from build123d import *

# Parameters (mm, degrees)
BOX_W          = 3.2
BOX_H          = 4.2
BOX_DEPTH      = 5
CYLINDER_R     = 4
CYLINDER_DEPTH = 10


with BuildPart() as obj1:
    # Box → Box (new body)
    with BuildSketch(Plane(origin=(-1.6, -2.1, 5), x_dir=(1, 0, 0), z_dir=(0, 0, 1))):
        with Locations((1.6, 2.1)):
            Rectangle(BOX_W, BOX_H)
    extrude(amount=BOX_DEPTH)


with BuildPart() as obj2:
    # Cylinder → Cylinder (new body)
    with BuildSketch(Plane.XY):
        Circle(CYLINDER_R)
    extrude(amount=CYLINDER_DEPTH)


with BuildPart() as obj3:
    # Sphere → Sphere (revolve)
    with BuildSketch(Plane.XZ):
        with BuildLine():
            ThreePointArc((0, -5), (5, 0), (0, 5))
            Line((0, 5), (0, -5))
        make_face()
    revolve(axis=Axis((0, 0, 0), (0, 0, 1)))

    # Fusion: union obj2
    add(obj2.part)

    # Cut: cut obj1
    add(obj1.part, mode=Mode.SUBTRACT)


solid = obj3.part
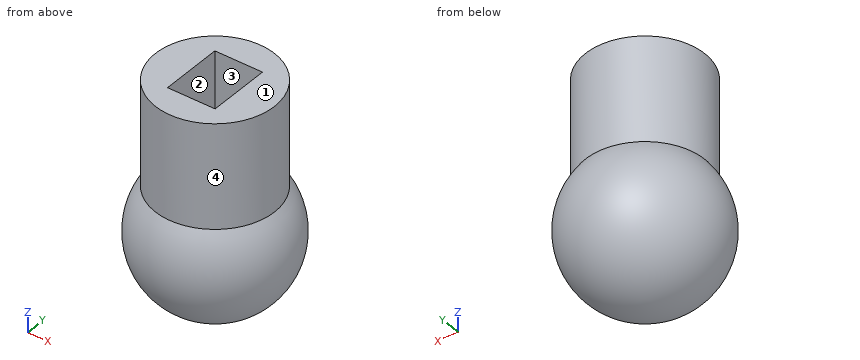
Could you check a few things on this model? Use its own coordinates, in mm. Face numbers are marked on the shaded views. Give positions to 0.01 mm unless a question says otherwise; leave off trailing zeros. Write each loop counter-clockwise with the first axis right and the second up, starting at its lowest first coordinate (ties: lowest second). Pieces come first, ordered by that corner, then holes. Notation, with made-up numbers: (-38, 41.5) - (16, 41.5) arc R13 ccw to (16, 64.5) - close; hole circle Ø2 at (-30.75, 88.25). An arc over 180 degrees is marked (long way). Use CSV: the item, a comma, the result in double quotes. Start each with the question number.
Item 1: I'm going to push flat-ended pins straight in: pin 1 (1.6 mm diameter, centred on x = 0, z = 6.5, fed in from +Y); pin 2 (5 mm diameter, centred on y = 0.5, z = 6, fed in from +X); pin 3 (1.6 mm diameter, centred on x = -0.5, z = 7.5, fed in from -Y); pin 4 (3.5 mm diameter, centred on x = 0, y = 0, fed in from +Z). Where does each tip first touch, or does it pass through?
Item 2: I want a section at B-B, the plane z = 6.75. Please give me the cut outline in (x, y), then the cut area to 3 significant figures.
Item 3: I want a section at D-D, the plane z = 0. Please give me the cut outline in (x, y), then the cut area to 3 significant figures.
Item 4: If I drill on line 1 along Y through (x, z) = (1.5, 9); line 2 along Y through (x, z) = (0, 6.75); line 3 along X through (y, z) = (1, 9.75), over which ranges is the centre line in solid material (lowest first)?
Item 5: I want a section at A-A, the plane y = 0. Please give me the cut outline in (x, z).
Item 6: If we mould it in two halves opening along X, with no side actions, what happens to the marked faces 1, 2, 3 and 4? For each: pulls with the +X half, pulls with the -X half, needs draft (parallel to the pull), parting line crosses it, or undercut.
Item 7: I want a section at C-C, the plane x = 0. Please give me the cut outline in (y, z).
Findings:
1,pin 1,"stops at y = 4"
1,pin 2,"stops at x = 4"
1,pin 3,"stops at y = -4"
1,pin 4,"stops at z = 10"
2,outline,"circle Ø8 at (0, 0); hole (-1.6, -2.1) - (1.6, -2.1) - (1.6, 2.1) - (-1.6, 2.1) - close"
2,area,"36.8 mm2"
3,outline,"circle Ø10 at (0, 0)"
3,area,"78.5 mm2"
4,line 1,"y = -3.71 to -2.1, 2.1 to 3.71"
4,line 2,"y = -4 to -2.1, 2.1 to 4"
4,line 3,"x = -3.87 to -1.6, 1.6 to 3.87"
5,outline,"(-4, 3) arc R5 ccw (long way) to (4, 3) - (4, 10) - (1.6, 10) - (1.6, 5) - (-1.6, 5) - (-1.6, 10) - (-4, 10) - close"
6,face 1,"needs draft"
6,face 2,"undercut"
6,face 3,"undercut"
6,face 4,"parting line crosses it"
7,outline,"(-4, 3) arc R5 ccw (long way) to (4, 3) - (4, 10) - (2.1, 10) - (2.1, 5) - (-2.1, 5) - (-2.1, 10) - (-4, 10) - close"
